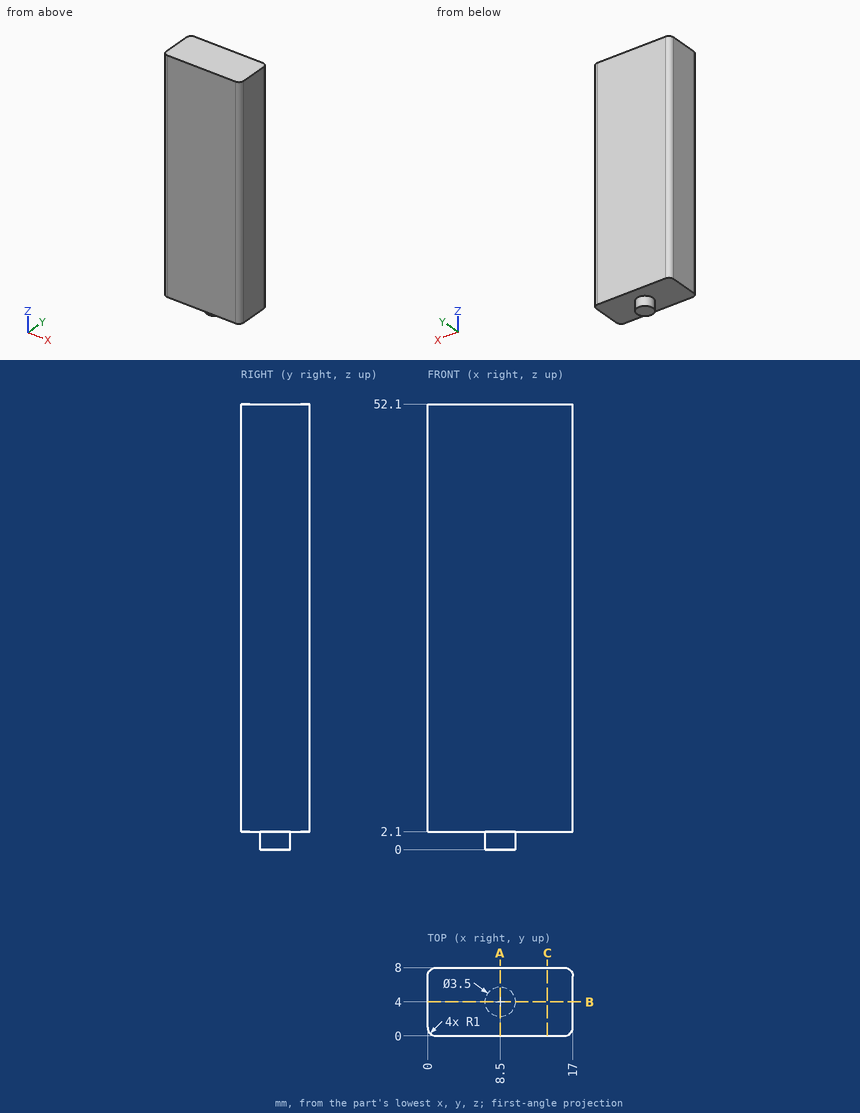
For this review, use the dimensioned drawing (mm, ordinates from the lowest corner) and the shaded views. Give positions to 0.01 mm unless a question says otherwise; leave off trailing zeros. Order: outer loops, then holes, each group sorted by start corner. A loop starts at its lowest first (then second) coordinate and runs counter-clockwise, first axis right, second up. Notation, with made-up numbers: (-13.75, 43.5) - (5.25, 43.5) arc R11 ccw to (5.25, 50.5) - close; hole circle Ø6 at (-17, 89.5). An arc over 180 degrees is marked (long way). Write item = value, one per line. Start each with the question number.
Q1. We need section C-C on x = 14. State the section outline as (y, z) points.
Q2. To check wall thickness, follow L1, parallel to Z at x = 3.25, y = 7.5; L2, parallel to X at y = 7.25, z = 48; L3, parallel to Y at x = 16.5, z = 8. State the ranges of each line that lie inside material, in increasing order. Write a range as from..to.
Q3. We need section B-B on y = 4. State the section outline as (x, z) points.
Q4. We need section A-A on x = 8.5. State the section outline as (y, z) points, plus the area to 3 significant figures.
Q5. Clearance check with a flat-ended pin moving along its axis: pin 1 Ø3 at (x, y) = (15.5, 4.5) entering from -Z. State where the tip first meets the part, or that it passes through.
Working result:
q1.outline = (0, 2.1) - (8, 2.1) - (8, 52.1) - (0, 52.1) - close
q2.L1 = 2.1..52.1
q2.L2 = 0.03..16.97
q2.L3 = 0.13..7.87
q3.outline = (0, 2.1) - (6.75, 2.1) - (6.75, 0) - (10.25, 0) - (10.25, 2.1) - (17, 2.1) - (17, 52.1) - (0, 52.1) - close
q4.outline = (0, 2.1) - (2.25, 2.1) - (2.25, 0) - (5.75, 0) - (5.75, 2.1) - (8, 2.1) - (8, 52.1) - (0, 52.1) - close
q4.area = 407 mm²
q5.pin_1 = 2.1
